from build123d import *

# Parameters (mm, degrees)
BOSS_EXTRUDE1_DEPTH = 61.2
SKETCH3_R           = 1.95
CUT_EXTRUDE1_DEPTH  = 2


with BuildPart() as part:
    # Sketch2 → Boss-Extrude1 (new body)
    with BuildSketch(Plane(origin=(0, 0, 0), x_dir=(0, 0, -1), z_dir=(1, 0, 0))):
        with BuildLine():
            Line((0, 0), (-10, 0))
            ThreePointArc((-10, 0), (-29, 19), (-48, 0))
            Line((-48, 0), (-60, 0))
            ThreePointArc((-60, 0), (-76.2, 16.2), (-92.4, 0))
            Line((-92.4, 0), (-102.4, 0))
            Line((-102.4, 0), (-102.4, 2))
            Line((-102.4, 2), (-94.289776118, 2))
            ThreePointArc((-94.289776118, 2), (-76.2, 18.2), (-58.110223882, 2))
            Line((-58.110223882, 2), (-49.90454496, 2))
            ThreePointArc((-49.90454496, 2), (-29, 21), (-8.09545504, 2))
            Line((-8.09545504, 2), (0, 2))
            Line((0, 2), (0, 0))
        make_face()
    extrude(amount=BOSS_EXTRUDE1_DEPTH)

    # Sketch3 → Cut-Extrude1 (cut)
    with BuildSketch(Plane(origin=(0, 2, 0), x_dir=(1, 0, 0), z_dir=(0, 1, 0))):
        with Locations(Location((12.24, -3.93, 0), (0, 0, 270))):
            Circle(SKETCH3_R)
        with Locations(Location((24.48, -3.93, 0), (0, 0, 270))):
            Circle(SKETCH3_R)
        with Locations(Location((36.72, -3.93, 0), (0, 0, 270))):
            Circle(SKETCH3_R)
        with Locations(Location((48.96, -3.93, 0), (0, 0, 270))):
            Circle(SKETCH3_R)
        with Locations(Location((12.24, -54.007384421, 0), (0, 0, 270))):
            Circle(SKETCH3_R)
        with Locations(Location((24.48, -54.007384421, 0), (0, 0, 270))):
            Circle(SKETCH3_R)
        with Locations(Location((36.72, -54.007384421, 0), (0, 0, 270))):
            Circle(SKETCH3_R)
        with Locations(Location((48.96, -54.007384421, 0), (0, 0, 270))):
            Circle(SKETCH3_R)
        with Locations(Location((12.24, -98.47, 0), (0, 0, 270))):
            Circle(SKETCH3_R)
        with Locations(Location((24.48, -98.47, 0), (0, 0, 270))):
            Circle(SKETCH3_R)
        with Locations(Location((36.72, -98.47, 0), (0, 0, 270))):
            Circle(SKETCH3_R)
        with Locations(Location((48.96, -98.47, 0), (0, 0, 270))):
            Circle(SKETCH3_R)
    extrude(amount=-CUT_EXTRUDE1_DEPTH, mode=Mode.SUBTRACT)


solid = part.part
Work out the finished part from the listing and answer in its coordinate system (mm). A direction names the side the tool comes from. Round coordinates to 2 decimals unless told otherwise and drop trailing zeros. Loops run counter-clockwise (first coordinate to the right, second up) from the corner with the lowest first, then second, coordinate; pieces in that order, holes last. Notation, with made-up numbers: (-27.5, -29.5) - (22.5, -29.5) arc R26 ccw to (22.5, 3.5) - close; hole circle Ø7 at (29, 60.5). An arc over 180 degrees is marked (long way). Use one line per item in the form item = value. Start each with the question number.
(1) Determine the mould class of faces 1 (the face through (38.364, 1.014, 4.978)), 2 (the face through (0, 10, 47)), 3 (the face through (30, 2, 98)) for opening direction X: +X half, -X half, draft (parallel to the pull), parting line (faces both ways), or undercut.
(2) Find section B-B on z = 98.47. Determine the outline of the cut face in (x, y).
(3) Find section A-A on x = 36.72. Determine the outline of the cut face in (y, z).
(4) Find section D-D on x = 21. Determine the outline of the cut face in (y, z).
(5) Find section C-C on y = 13.5. Determine the outline of the cut face in (x, z).
(6) Flat-ended cylindrical pins translate along their axes: P1, Ø5, axis at x = 33, y = 11, coming from the -Z side; P2, Ø2.5, axis at x = 36.72, z = 3.93, coming from the +Y side; P3, Ø5, axis at x = 26, y = 9, coming from the +Z side; P4, Ø8, axis at x = 30.5, y = 17, coming from the -Z side. Find the tip coordinate at first contact, or state that the pin passes through.
(7) Which of the six approach directions +Z, -Z, +X, -X, +Y, -Y give full straight-line access (tool end or side, diameter ignored) to faces 4 (the face through (30, 2, 54)), 5 (the face through (38.364, 1.014, 99.518)), 6 (the face through (30, 2, 4))?
(8) Consider line 1 (X direction, y = 1.3, z = 3.93); line 2 (Z direction, x = 33.5, y = 1.25); line 3 (Z direction, x = 25, y = 5.75). Determine where each line is inside the solid, lowest interval first.
Answer list:
q1.face_1 = undercut
q1.face_2 = -X half
q1.face_3 = draft
q2.outline = (0, 0) - (10.29, 0) - (10.29, 2) - (0, 2) - close; (14.19, 0) - (22.53, 0) - (22.53, 2) - (14.19, 2) - close; (26.43, 0) - (34.77, 0) - (34.77, 2) - (26.43, 2) - close; (38.67, 0) - (47.01, 0) - (47.01, 2) - (38.67, 2) - close; (50.91, 0) - (61.2, 0) - (61.2, 2) - (50.91, 2) - close
q3.outline = (0, 0) - (2, 0) - (2, 1.98) - (0, 1.98) - close; (0, 5.88) - (2, 5.88) - (2, 8.1) arc R21 ccw to (2, 49.9) - (2, 52.06) - (0, 52.06) - (0, 48) arc R19 cw to (0, 10) - close; (0, 55.96) - (2, 55.96) - (2, 58.11) arc R18.2 ccw to (2, 94.29) - (2, 96.52) - (0, 96.52) - (0, 92.4) arc R16.2 cw to (0, 60) - close; (0, 100.42) - (2, 100.42) - (2, 102.4) - (0, 102.4) - close
q4.outline = (0, 0) - (2, 0) - (2, 8.1) arc R21 ccw to (2, 49.9) - (2, 58.11) arc R18.2 ccw to (2, 94.29) - (2, 102.4) - (0, 102.4) - (0, 92.4) arc R16.2 cw to (0, 60) - (0, 48) arc R19 cw to (0, 10) - close
q5.outline = (0, 12.91) - (61.2, 12.91) - (61.2, 15.63) - (0, 15.63) - close; (0, 42.37) - (61.2, 42.37) - (61.2, 45.09) - (0, 45.09) - close; (0, 63.99) - (61.2, 63.99) - (61.2, 67.25) - (0, 67.25) - close; (0, 85.15) - (61.2, 85.15) - (61.2, 88.41) - (0, 88.41) - close
q6.P1 = 9.8
q6.P2 = through
q6.P3 = 93.2
q6.P4 = 12.51
q7.face_4 = +X, -X, +Y
q7.face_5 = +Y, -Y
q7.face_6 = -Z, +X, -X, +Y
q8.line_1 = 0 to 10.29, 14.19 to 22.53, 26.43 to 34.77, 38.67 to 47.01, 50.91 to 61.2
q8.line_2 = 0 to 10.04, 47.96 to 60.05, 92.35 to 102.4
q8.line_3 = 8.8 to 10.89, 47.11 to 49.2, 58.93 to 61.05, 91.35 to 93.47
